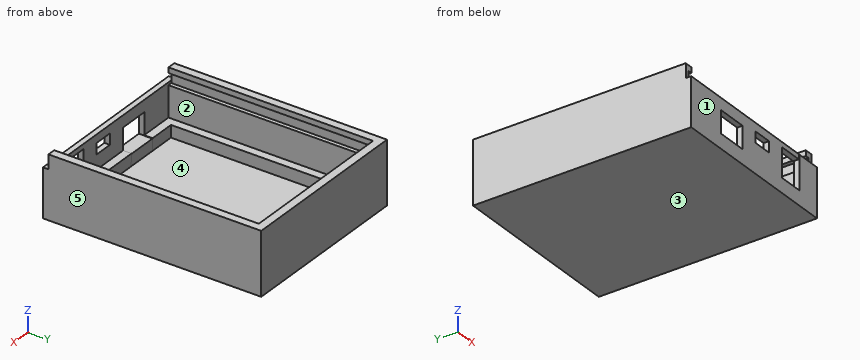
Autodesk Fusion 360 part; units mm, degrees
sketch "Esquisse1" plane through (0, 0, 0) normal (0, 0, 1) x (1, 0, 0)
  line L0 (0, 0) -> (53.5, 0)
  line L1 (53.5, 0) -> (53.5, 66.4)
  line L2 (0, 66.4) -> (0, 0)
  line L3 (41.3, 0) -> (50.3, 0)
  line L4 (50.3, 0) -> (50.3, -5.2)
  line L5 (50.3, -5.2) -> (41.3, -5.2)
  line L6 (41.3, -5.2) -> (41.3, 0)
  line L7 (11.5, 0) -> (18.8, 0)
  line L8 (18.8, 0) -> (18.8, -1.2)
  line L9 (18.8, -1.2) -> (11.5, -1.2)
  line L10 (11.5, -1.2) -> (11.5, 0)
  line L11 (53.5, 66.4) -> (51.2, 66.4) construction
  line L12 (51.2, 66.4) -> (49.0195, 69)
  line L13 (49.0195, 69) -> (14.9195, 69)
  line L14 (12.5, 66.4) -> (14.9195, 69)
  line L15 (53.5, 66.4) -> (51.2, 66.4)
  line L16 (12.5, 66.4) -> (0, 66.4)
  line L17 (41.3, 0) -> (49.9, 0)
  line L18 (11.5, 0) -> (18.8, 0)
  line L19 (0, 33.2) -> (53.5, 33.2) construction
  line L20 (26.75, 0) -> (26.75, 33.2) construction
  line L21 (0, 66.4) -> (0, 68.7) construction
  line L22 (0, 68.7) -> (53.5, 68.7) construction
  line L23 (53.5, 68.7) -> (53.5, 66.4) construction
  line L24 (-3, 72) -> (56.5, 72)
  line L25 (56.5, 72) -> (56.5, -3)
  line L26 (56.5, -3) -> (-3, -3)
  line L27 (-3, -3) -> (-3, 72)
  line L28 (-6, 75) -> (59.5, 75)
  line L29 (59.5, 75) -> (59.5, -5)
  line L30 (59.5, -5) -> (-6, -5)
  line L31 (-6, -5) -> (-6, 75)
  line L32 (26.75, 75) -> (26.75, -5) construction
  line L33 (11.5, -1.2) -> (11.5, -5)
  line L34 (18.8, -1.2) -> (18.8, -5)
  line L35 (15.15, 0) -> (15.15, -5) construction
  line L36 (9.55, 0) -> (20.75, 0)
  line L37 (20.75, 0) -> (20.75, -5)
  line L38 (20.75, -5) -> (9.55, -5)
  line L39 (9.55, -5) -> (9.55, 0)
  line L40 (15.15, 0) -> (15.15, -5) construction
  line L41 (-3, -3) -> (-6, -3)
  line L42 (56.5, -3) -> (59.5, -3)
  dimension "d1" = 66.4
  dimension "d13" = 53.5
  dimension "d14" = 3.2
  dimension "d15" = 9
  dimension "d16" = 5.2
  dimension "d17" = 11.5
  dimension "d18" = 7.3
  dimension "d19" = 1.2
  dimension "d21" = 2.3
  dimension "d22" = 38.7
  dimension "d25" = 34.1
  dimension "d43" = 3
  dimension "d44" = 3
  dimension "d45" = 3
  dimension "d46" = 3
  dimension "d47" = 3
  dimension "d48" = 3
  dimension "d52" = 11.2
extrude "Extrusion6" add sketch "Esquisse1" along normal blind 1 contours L0 L1 L2 L3 L7 L12 L13 L14 L15 L16 L17 L18 L36
extrude "Extrusion7" add sketch "Esquisse1" along normal blind 5.5 draft 1 contours L0 L1 L2 L4 L12 L13 L14 L15 L16 L24 L25 L26 L27 L39 | L0 L6 L26 L37
extrude "Extrusion8" add sketch "Esquisse1" along normal blind 23 contours L24 L25 L27 L28 L29 L31 L41 L42
extrude "Extrusion9" add sketch "Esquisse1" along normal blind 4.5 contours L0 L10 L26 L33 L36 L39 | L0 L7 L8 L9 L10 L18 L36 | L26 L30 L33 L38 L39 | L0 L8 L26 L34 L36 L37 | L9 L26 L33 L34 | L26 L30 L33 L34 L38 | L26 L30 L34 L37 L38 | L0 L3 L4 L6 L17 L26 | L4 L6 L26 L30
extrude "Extrusion10" add sketch "Esquisse1" along normal blind 17.8 contours L26 L30 L31 L39 L41 | L6 L26 L30 L37 | L4 L26 L29 L30 L42
sketch "Esquisse2" plane through (-3, 0, 0) normal (1, 0, 0) x (0, 1, 0)
  line L0 (-3, 5.5) -> (72, 5.5)
  line L1 (72, 5.5) -> (72, 23)
  line L2 (72, 23) -> (-3, 23)
  line L3 (-3, 23) -> (-3, 17.8)
  line L4 (-3, 17.8) -> (-3, 5.5)
  line L5 (-3, 23) -> (75, 23) construction
  line L6 (-3, 21) -> (72.5, 21)
  line L7 (72.5, 21) -> (72.5, 16.8)
  line L8 (72.5, 16.8) -> (-3, 16.8)
  line L9 (-3, 16.8) -> (-3, 21)
  dimension "d65" = 2
  dimension "d66" = 4.2
  dimension "d67" = 75.5
extrude "Extrusion11" cut sketch "Esquisse2" against normal blind 1.5 contours L1 L3 L4 L6 L8 L9
sketch "Esquisse3" plane through (56.5, 0, 0) normal (-1, 0, 0) x (0, -1, 0)
  line L0 (-72, 5.5) -> (3, 5.5)
  line L1 (3, 5.5) -> (3, 17.8)
  line L2 (3, 17.8) -> (3, 23)
  line L3 (3, 23) -> (-72, 23)
  line L4 (-72, 23) -> (-72, 5.5)
  line L5 (-72, 23) -> (3, 23) construction
  line L6 (-72, 21) -> (3, 21)
  line L7 (3, 21) -> (3, 16.8)
  line L8 (3, 16.8) -> (-72, 16.8)
  line L9 (-72, 16.8) -> (-72, 21)
  dimension "d70" = 4.2
  dimension "d71" = 2
extrude "Extrusion12" cut sketch "Esquisse3" against normal blind 1.5 contours L1 L2 L4 L6 L7 L8 L9
sketch "Esquisse4" plane through (0, 72, 0) normal (0, -1, 0) x (1, 0, 0)
  line L0 (-3, 5.5) -> (56.5, 5.5)
  line L1 (56.5, 5.5) -> (56.5, 16.8)
  line L2 (56.5, 16.8) -> (58, 16.8)
  line L3 (58, 16.8) -> (58, 21)
  line L4 (58, 21) -> (56.5, 21)
  line L5 (56.5, 21) -> (56.5, 23)
  line L6 (56.5, 23) -> (-3, 23)
  line L7 (-3, 23) -> (-3, 21)
  line L8 (-3, 21) -> (-4.5, 21)
  line L9 (-4.5, 21) -> (-4.5, 16.8)
  line L10 (-4.5, 16.8) -> (-3, 16.8)
  line L11 (-3, 16.8) -> (-3, 5.5)
  line L12 (-4.5, 21) -> (58, 21)
  line L13 (58, 21) -> (58, 16.8)
  line L14 (58, 16.8) -> (-4.5, 16.8)
  line L15 (-4.5, 16.8) -> (-4.5, 21)
extrude "Extrusion13" add 2 faces at (47.2738, -2.0524, 4.5) (16.9905, -1.0262, 4.5) along direction (0, 0, 1) blind 0.8
sketch "Esquisse5" plane through (0, -3, 0) normal (0, 1, 0) x (-1, 0, 0)
  line L0 (-41.3, 5.5) -> (-20.75, 5.5)
  line L1 (-20.75, 5.5) -> (-20.75, 17.8)
  line L2 (-20.75, 17.8) -> (-41.3, 17.8)
  line L3 (-41.3, 17.8) -> (-41.3, 5.5)
  line L4 (-60.0312, 14.8) -> (4.9812, 14.8) construction
  line L5 (-50, 16) -> (-41.3, 16) construction
  line L6 (-20.75, 13.5) -> (-9.5, 13.5) construction
  line L7 (-41.3, 5.5) -> (-51, 5.5) construction
  line L8 (-51, 5.5) -> (-20.75, 5.5) construction
  line L9 (-9.284, 5.5) -> (-20.75, 5.5) construction
  line L10 (-50, 16) -> (-41.3, 16)
  line L11 (-41.3, 16) -> (-41.3, 17.8)
  line L12 (-41.3, 17.8) -> (-50, 17.8)
  line L13 (-50, 17.8) -> (-50, 16)
  line L14 (-20.75, 17.8) -> (-9.5, 17.8)
  line L15 (-9.5, 17.8) -> (-9.5, 13.5)
  line L16 (-9.5, 13.5) -> (-20.75, 13.5)
  line L17 (-20.75, 13.5) -> (-20.75, 17.8)
  line L18 (-27.525, 14.8) -> (-34.525, 14.8)
  line L19 (-34.525, 14.8) -> (-34.525, 10.8)
  line L20 (-34.525, 10.8) -> (-27.525, 10.8)
  line L21 (-27.525, 10.8) -> (-27.525, 14.8)
  line L22 (-20.75, 17.8) -> (-41.3, 17.8) construction
  line L23 (-41.3, 17.8) -> (-41.3, 5.5) construction
  line L24 (-41.3, 5.5) -> (-20.75, 5.5) construction
  line L25 (-20.75, 5.5) -> (-20.75, 17.8) construction
  line L26 (-31.025, 14.8) -> (-31.025, 10.8) construction
  line L27 (-31.025, 17.8) -> (-31.025, 5.5) construction
  dimension "d76" = 10.5
  dimension "d78" = 8
  dimension "d81" = 7
  dimension "d82" = 4
extrude "Extrusion14" add sketch "Esquisse5" against normal blind 2 contours L3 L10 L11 L12 L13 | L1 L14 L15 L16 L17
extrude "Extrusion16" cut sketch "Esquisse5" against normal blind 2 contours L18 L19 L20 L21
extrude "Extrusion17" cut sketch "Esquisse4" against normal blind 1 contours L2 L3 L4 L8 L9 L10 L12 L13 L14 L15
extrude "Extrusion19" cut 1 faces at (47.1, -3.6667, 16) along direction (0, 0, -1) blind 3
equation "d1 = longc1"
equation "longc1 = longueur Carte"
equation "largc1 = largueur Carte"
equation "diffdepH = 2.5 mm"
equation "epchar = 11 mm"
equation "depconn = 1.2 mm"
equation "depchar = 5.2 mm"
equation "larchar = 9 mm"
equation "larconn = 7.3 mm"
equation "distborconn = 11.5 mm"
equation "distborchar = 3.2 mm"
equation "diffdepD = 2.3 mm"
equation "d13 = largc1"
equation "d14 = distborchar"
equation "d15 = larchar"
equation "d16 = depchar"
equation "d17 = distborconn"
equation "d18 = larconn"
equation "d19 = depconn"
equation "largdep = 34.2 mm"
equation "d21 = diffdepD"
equation "epC = 4.5 mm"
equation "epconn = 2.5 mm"
equation "diffCB = espace entre bordure et carte"
equation "d43 = diffCB"
equation "d44 = diffCB"
equation "d45 = diffCB"
equation "d46 = diffCB"
equation "d47 = epB"
equation "d48 = epB"
equation "epB = 3 mm"
equation "Lpu = largeur de l'embout USB-c"
equation "Hpu = Hauteur de l'embout USB-c"
equation "d52 = Lpu"
equation "d55 = 1 mm + epC"
equation "HB = Hauteur Boite"
equation "epV = 3.2 mm"
equation "d59 = HB"
equation "d61 = epC"
equation "d63 = HB - 2 mm - epV"
equation "d66 = epV + 1 mm"
equation "d67 = 78.000001 mm - 2.5 mm"
equation "d70 = epV + 1 mm"
equation "d76 = HC"
equation "HC = hauteur del'embout chargeur"
equation "d78 = Hpu"
equation "longpin = 3 mm"
The listing builds one solid part. Answer for the finished solid, in the listing's coordinates (mm). Face numbers are marked on the shaded views. A direction names the side the tool comes from. Give positions to 0.01 mm unless a question says otherwise; leave off trailing zeros. Write each loop counter-clockwise with the first axis right and the second up, starting at its lowest first coordinate (ties: lowest second). Pieces come first, ordered by that corner, then holes.
1) Find the intervals of material crossed by L1, parallel to Y at x = 16, z = 17; L2, parallel to Y at x = -2.5, z = 8.5; L3, parallel to X at y = 9, z = 16.5, in increasing order.
2) Given P1, Ø0.6, axis at x = 56.5, y = -4, coming from the +Z side; P2, Ø8, axis at x = 10.5, y = 22, coming from the +Z side, each flat-ended and moving along its own axis, determine where each tip first touches the part or whether it passes through.
3) Section C-C (z = 20) is taken. Write down the section's boundary in (x, y), and give its area (3 significant figures).
4) Section D-D (y = 47.5) is taken. Write down the section's boundary in (x, z), and give its area (3 significant figures).
5) Section A-A (x = 18.5) is taken. Write down the section's boundary in (y, z), and give its area (3 significant figures).
6) A tool of negligible diameter and unlimited length cuts with its end or side. For the marked faces 1 and 2, from which of +Z, -Z, +X, -X, +Y, -Y can it reach the whole face along a straight path? Write none if from no direction.
7) For a pull along X with two mould halves and no side action, classify the marked faces 3, 4 and 5 as pulls with the +X half, pulls with the -X half, needs draft (parallel to the pull), parting line crosses it, or undercut.
8) Section B-B (z = 7.5) is taken. Write down the section's boundary in (x, y).
Response:
1. L1: y = -5 to -3, 73 to 75
1. L2: y = -5 to -3, 72 to 75
1. L3: x = -6 to -3, 56.5 to 59.5
2. P1: stops at z = 17.8
2. P2: stops at z = 1
3. outline: (-6, -3) - (-4.5, -3) - (-4.5, 73) - (58, 73) - (58, -3) - (59.5, -3) - (59.5, 75) - (-6, 75) - close
3. area: 359 mm2
4. outline: (-6, 0) - (59.5, 0) - (59.5, 23) - (56.5, 23) - (56.5, 21) - (58, 21) - (58, 16.8) - (56.5, 16.8) - (56.5, 5.5) - (53.4, 5.5) - (53.48, 1) - (0.02, 1) - (0.1, 5.5) - (-3, 5.5) - (-3, 16.8) - (-4.5, 16.8) - (-4.5, 21) - (-3, 21) - (-3, 23) - (-6, 23) - close
4. area: 212 mm2
5. outline: (-5, 0) - (75, 0) - (75, 23) - (72, 23) - (72, 21) - (73, 21) - (73, 16.8) - (72, 16.8) - (72, 5.5) - (68.9, 5.5) - (68.98, 1) - (0, 1) - (0, 5.3) - (-5, 5.3) - close; (-5, 13.5) - (-3, 13.5) - (-3, 17.8) - (-5, 17.8) - close
5. area: 186 mm2
6. face 1: +Z, -Z, +X, -X, -Y
6. face 2: +Z
7. face 3: needs draft
7. face 4: undercut
7. face 5: pulls with the +X half
8. outline: (-6, -5) - (9.55, -5) - (9.55, -3) - (-3, -3) - (-3, 72) - (56.5, 72) - (56.5, -3) - (50.3, -3) - (50.3, -5) - (59.5, -5) - (59.5, 75) - (-6, 75) - close; (20.75, -5) - (41.3, -5) - (41.3, -3) - (20.75, -3) - close
